Source: CAD feature listing. Evaluate the final solid. Frame: model axes, mm. A direction names the side the tool comes from. Coordinates: 2 decimals unless noted, no trailing zeros. Loops run counter-clockwise (first coordinate to the right, second up) from the corner with the lowest first, then second, coordinate; pieces in that order, holes last.
Item 1: Section query D-D, the plane x = 10. Return the cut outline in (y, z).
Item 2: Line query: probe 1 along X at (y, z) = (7.75, 0.65); probe 2 along Y at (x, z) = (67, 1.05); probe 3 along Y at (x, z) = (10, 2). Output: solid intervals per line, ascending.
Item 3: Reachability of faces 5 (the cylindrical face through (20.296, -0.307, 1.521)), 6 (the flat face through (48, 15, 1)) from +Z, -Z, +X, -X, +Y, -Y: full face, straight path, thin tool, end or side. Return the list, or none.
Item 4: Pull-direction query (Y, two-part tool) for faces 1 (the cylindrical face through (14.77, 9, 1.48)), 2 (the cylindrical face through (40.526, 8.852, 1.479)), 3 (the flat face through (37, 8, 0)), 4 (the flat face through (47, 0, 1)); classes: +Y half, -Y half, draft (parallel to the pull), parting line (faces both ways), or undercut.
Item 5: Section query A-A, the plane x = 42. Return the cut outline in (y, z).
Item 6: Section query C-C, the plane z = 0.55. Return the cut outline in (x, y), then the cut area to 3 significant figures.
Item 7: Pin query (flat end, axial travel): pin 1 Ø1 at (x, z) = (54.5, 0.5) entering from -Y; pin 2 Ø1.5 at (x, z) = (47, 1) entering from +Y; pin 3 Ø1.5 at (y, z) = (13, 1.5) entering from +X; pin 4 Ø5 at (x, y) = (42, 7.5) entering from +Z. Return the tip coordinate at first contact, or that it passes through.
Item 8: Section query B-B, the plane y = 7.5. Return the cut outline in (x, z), then the cut area to 4 significant figures.
```python
from build123d import *

# Parameters (mm, degrees)
SKETCH1_R           = 5
SKETCH1_R_2         = 2
BOSS_EXTRUDE1_DEPTH = 3
FILLET2_R           = 4


with BuildPart() as part:
    # Sketch1 → Boss-Extrude1 (new body)
    with BuildSketch(Plane.XY):
        with BuildLine():
            Line((20, 0), (77, 0))
            Line((77, 0), (77, 15))
            Line((77, 15), (20, 15))
            ThreePointArc((20, 15), (-2.5, 7.5), (20, 0))
        make_face()
        with Locations((10, 7.5)):
            Circle(SKETCH1_R, mode=Mode.SUBTRACT)
        with Locations((67, 7.5)):
            Circle(SKETCH1_R_2, mode=Mode.SUBTRACT)
        with Locations((42, 7.5)):
            Circle(SKETCH1_R_2, mode=Mode.SUBTRACT)
    extrude(amount=BOSS_EXTRUDE1_DEPTH)

    # Fillet2
    fillet2_edges = [part.edges().sort_by_distance(p)[0] for p in [
        (20, 15, 1.5),
        (77, 15, 1.5),
        (77, 0, 1.5),
        (20, 0, 1.5),
    ]]
    fillet(fillet2_edges, radius=FILLET2_R)


solid = part.part
```
Verdict:
1. outline: (-5, 0) - (2.5, 0) - (2.5, 3) - (-5, 3) - close; (12.5, 0) - (20, 0) - (20, 3) - (12.5, 3) - close
2. probe 1: x = -2.5 to 5.01, 14.99 to 40.02, 43.98 to 65.02, 68.98 to 77
2. probe 2: y = 0 to 5.5, 9.5 to 15
2. probe 3: y = -5 to 2.5, 12.5 to 20
3. face 5: +Z, -Z, +X, -Y
3. face 6: +Z, -Z, +X, +Y
4. face 1: undercut
4. face 2: undercut
4. face 3: draft
4. face 4: -Y half
5. outline: (0, 0) - (5.5, 0) - (5.5, 3) - (0, 3) - close; (9.5, 0) - (15, 0) - (15, 3) - (9.5, 3) - close
6. outline: (18.96, -1.21) arc R4 cw to (21.83, 0) - (73, 0) arc R4 ccw to (77, 4) - (77, 11) arc R4 ccw to (73, 15) - (21.83, 15) arc R4 cw to (18.96, 16.21) arc R12.5 ccw (long way) to start; hole circle Ø10 at (10, 7.5); hole circle Ø4 at (42, 7.5); hole circle Ø4 at (67, 7.5)
6. area: 1,210 mm2
7. pin 1: stops at y = 0
7. pin 2: stops at y = 15
7. pin 3: stops at x = 76.8
7. pin 4: stops at z = 3
8. outline: (-2.5, 0) - (5, 0) - (5, 3) - (-2.5, 3) - close; (15, 0) - (40, 0) - (40, 3) - (15, 3) - close; (44, 0) - (65, 0) - (65, 3) - (44, 3) - close; (69, 0) - (77, 0) - (77, 3) - (69, 3) - close
8. area: 184.5 mm2
